```python
from build123d import *

# Parameters (mm, degrees)
F0_W      = 355.6000034809
F0_H      = 279.4000034809
F1_DEPTH  = 304.8
F2_R      = 104.14
F3_DEPTH  = 12.6999982595
F4_R      = 88.9
F4_R_2    = 20.32
F5_DEPTH  = 12.7
F6_R      = 88.9
F6_R_2    = 20.32
F7_DEPTH  = 12.7
F9_DEPTH  = 12.7
F11_DEPTH = 12.7


with BuildPart() as f1:
    # F0 (on Top) → F1 (new body)
    with BuildSketch(Plane.XY):
        Polygon((0, 304.8), (0, 0), (22.8952505992, 0), (368.3, 0), (381, 0), (381, 304.8), (368.3, 304.8), (22.8952505992, 304.8), align=None)
        with Locations((190.5, 152.4)):
            Rectangle(F0_W, F0_H, mode=Mode.SUBTRACT)
        Polygon((22.8952505992, 0), (0, 0), (228.6, -152.4), (381, -152.4), (381, 0), (368.3, 0), (368.3, -139.7), (232.4452505992, -139.7), align=None)
        Polygon((228.6, 457.2), (0, 304.8), (22.8952505992, 304.8), (232.4452505992, 444.5), (368.3, 444.5), (368.3, 304.8), (381, 304.8), (381, 457.2), align=None)
    extrude(amount=F1_DEPTH)

    # F2 (on face) → F3 (cut, through all)
    with BuildSketch(Plane(origin=(0, 0, 0), x_dir=(0, -1, 0), z_dir=(-1, 0, 0))):
        with Locations((-152.4, 152.4)):
            Circle(F2_R)
    extrude(amount=-F3_DEPTH, mode=Mode.SUBTRACT)

    # F4 (on face) → F5 (cut, through all)
    with BuildSketch(Plane(origin=(-140.6769230769, 211.0153846154, 0), x_dir=(-0.8320502943, -0.5547001962, 0), z_dir=(-0.5547001962, 0.8320502943, 0))):
        with Locations((-323.1656269998, 133.8491573491)):
            Circle(F4_R)
        with Locations((-224.529868778, 243.2757062301)):
            Circle(F4_R_2)
    extrude(amount=-F5_DEPTH, mode=Mode.SUBTRACT)

    # F6 (on face) → F7 (cut, through all)
    with BuildSketch(Plane(origin=(0, 0, 0), x_dir=(0.8320502943, -0.5547001962, 0), z_dir=(-0.5547001962, -0.8320502943, 0))):
        with Locations((154.0930071904, 133.8491573491)):
            Circle(F6_R)
        with Locations((55.4572489685, 243.2757062301)):
            Circle(F6_R_2)
    extrude(amount=-F7_DEPTH, mode=Mode.SUBTRACT)

    # F8 (on face) → F9 (join)
    with BuildSketch(Plane(origin=(0, 0, 0), x_dir=(1, 0, 0), z_dir=(0, 0, -1))):
        Polygon((381, -457.2), (381, 152.4), (228.6, 152.4), (0, 0), (0, -304.8), (228.6, -457.2), align=None)
    extrude(amount=F9_DEPTH)

    # F10 (on face) → F11 (join)
    with BuildSketch(Plane.XY.offset(304.8)):
        Polygon((381, -152.4), (381, 457.2), (228.6, 457.2), (0, 304.8), (0, 0), (228.6, -152.4), align=None)
    extrude(amount=F11_DEPTH)


solid = f1.part
```
Could you check a few things on this model? Use its own coordinates, in mm. A direction names the side the tool comes from. Coordinates: 2 decimals unless noted, no trailing zeros. Write each loop counter-clockwise with the first axis right and the second up, starting at its lowest first coordinate (ties: lowest second). Pieces come first, ordered by that corner, then holes. Notation, with made-up numbers: (28.5, 33.5) -> (74.5, 33.5) arc R21 cw to (74.5, 56.5) -> close; hole circle Ø5 at (3.5, 11). An arc over 180 degrees is marked (long way). One line per question, with ' | ' between items. Start each with the question number.
1. Please list where these lines run through material, in increasing order: line 1 along Y through (x, z) = (251.5, 96); line 2 along Z through (x, y) = (299.5, 359); line 3 along Y through (x, z) = (104.5, 45.5).
2. If we section it at A-A (z = 37): Please give me the cut outline in (x, y), and give its area (3 significant figures).
3. Will this pin go through, and if not, where does the flat tip stop? P1, Ø3, axis at y = 69.5, z = 105, coming from the -X side.
4. Thinking about a two-plate mould opening in Y: for faces 1 (the face through (198, 304.8, 150)), 2 (the face through (61.9, -41.267, 186.777)), 3 (the face through (306, 457.2, 150)), which applies, pulls with the +Y half, pulls with the -Y half, needs draft (parallel to the pull), parting line crosses it, or undercut?
5. If we section it at B-B (y = 152.4): Please give me the cut outline in (x, z).
6. For faces 4 (the face through (304, -152.4, 150)), 5 (the face through (232, 360, 304.8)), 6 (the face through (6.26, 235.04, 89.03)), which set-ups out of +Z, -Z, +X, -X, +Y, -Y let a thin tool reach every point of the face, with its end or its side?
7. If we section it at D-D (y = 89.5): Please give me the cut outline in (x, z), and give its area (3 significant figures).
Return value:
1) line 1: y = -152.4 to -139.7, 0 to 12.7, 292.1 to 304.8, 444.5 to 457.2 | line 2: z = -12.7 to 0, 304.8 to 317.5 | line 3: y = -69.67 to -54.4, 0 to 12.7, 292.1 to 304.8, 359.2 to 374.47
2) outline: (0, 0) -> (228.6, -152.4) -> (381, -152.4) -> (381, 457.2) -> (228.6, 457.2) -> (0, 304.8) -> close; hole (12.7, 12.7) -> (368.3, 12.7) -> (368.3, 292.1) -> (12.7, 292.1) -> close; hole (22.9, 0) -> (232.45, -139.7) -> (368.3, -139.7) -> (368.3, 0) -> close; hole (22.9, 304.8) -> (368.3, 304.8) -> (368.3, 444.5) -> (232.45, 444.5) -> close | area: 30,800 mm²
3) P1: stops at x = 368.3
4) face 1: undercut | face 2: pulls with the -Y half | face 3: pulls with the +Y half
5) outline: (0, -12.7) -> (381, -12.7) -> (381, 317.5) -> (0, 317.5) -> (0, 256.54) -> (12.7, 256.54) -> (12.7, 304.8) -> (368.3, 304.8) -> (368.3, 0) -> (12.7, 0) -> (12.7, 48.26) -> (0, 48.26) -> close
6) face 4: +Z, -Z, +X, -X, -Y | face 5: none | face 6: -X
7) outline: (0, -12.7) -> (381, -12.7) -> (381, 317.5) -> (0, 317.5) -> (0, 235.4) -> (12.7, 235.4) -> (12.7, 304.8) -> (368.3, 304.8) -> (368.3, 0) -> (12.7, 0) -> (12.7, 69.4) -> (0, 69.4) -> close | area: 15,300 mm²
